```python
from build123d import *

# Parameters (mm, degrees)
SKETCH1_R           = 28
BOSS_EXTRUDE1_DEPTH = 55
CUT_EXTRUDE1_DEPTH  = 35
SKETCH3_R           = 28
SKETCH3_R_2         = 20
BOSS_EXTRUDE2_DEPTH = 35
SKETCH4_R           = 29
BOSS_EXTRUDE3_DEPTH = 87.5


with BuildPart() as part:
    # Sketch1 → Boss-Extrude1 (new, symmetric)
    with BuildSketch(Plane(origin=(0, 0, 0), x_dir=(0, 0, -1), z_dir=(1, 0, 0))):
        with BuildLine():
            ThreePointArc((1633.779443993, -91.870179926), (1388.538518192, -287.439228591), (1079.911873115, -343.474560585))
            ThreePointArc((1079.911873115, -343.474560585), (1044.034822803, -322.026545424), (1040.331298925, -280.391656157))
            ThreePointArc((1040.331298925, -280.391656157), (1037.457004109, -237.066241511), (1001.77399927, -212.326065873))
            Line((1001.77399927, -212.326065873), (-8.291026647, -52.347482052))
            ThreePointArc((-8.291026647, -52.347482052), (-52.836618688, 4.158332074), (0, 53))
            Line((0, 53), (1402, 53))
            Line((1402, 53), (1609.372117166, -14))
            ThreePointArc((1609.372117166, -14), (1641.711266017, -46.623901593), (1633.779443993, -91.870179926))
        make_face()
        with Locations((1373, 19)):
            Circle(SKETCH1_R, mode=Mode.SUBTRACT)
    extrude(amount=BOSS_EXTRUDE1_DEPTH, both=True)

    # Sketch2 → Cut-Extrude1 (cut, symmetric)
    with BuildSketch(Plane(origin=(0, 0, 0), x_dir=(0, 0, -1), z_dir=(1, 0, 0))):
        with BuildLine():
            Line((1462.900269506, 33.323690028), (1249.391694757, -251.544855987))
            Line((1249.391694757, -251.544855987), (1001.77399927, -212.326065873))
            ThreePointArc((1001.77399927, -212.326065873), (1037.457004109, -237.066241511), (1040.331298925, -280.391656157))
            ThreePointArc((1040.331298925, -280.391656157), (1044.034822803, -322.026545424), (1079.911873115, -343.474560585))
            ThreePointArc((1079.911873115, -343.474560585), (1388.538518192, -287.439228591), (1633.779443993, -91.870179926))
            ThreePointArc((1633.779443993, -91.870179926), (1641.711266017, -46.623901593), (1609.372117166, -14))
            Line((1609.372117166, -14), (1462.900269506, 33.323690028))
        make_face()
    extrude(amount=CUT_EXTRUDE1_DEPTH, both=True, mode=Mode.SUBTRACT)

    # Sketch3 → Boss-Extrude2 (add, symmetric)
    with BuildSketch(Plane(origin=(0, 0, 0), x_dir=(0, 0, -1), z_dir=(1, 0, 0))):
        with Locations((1594, -61.578335551)):
            Circle(SKETCH3_R)
        with Locations((1083, -297.578335551)):
            Circle(SKETCH3_R_2)
    extrude(amount=BOSS_EXTRUDE2_DEPTH, both=True)

    # Sketch4 → Boss-Extrude3 (add, symmetric)
    with BuildSketch(Plane(origin=(0, 0, 0), x_dir=(0, 0, -1), z_dir=(1, 0, 0))):
        Circle(SKETCH4_R)
        with Locations((157, -14)):
            Circle(SKETCH4_R)
    extrude(amount=BOSS_EXTRUDE3_DEPTH, both=True)


solid = part.part
```
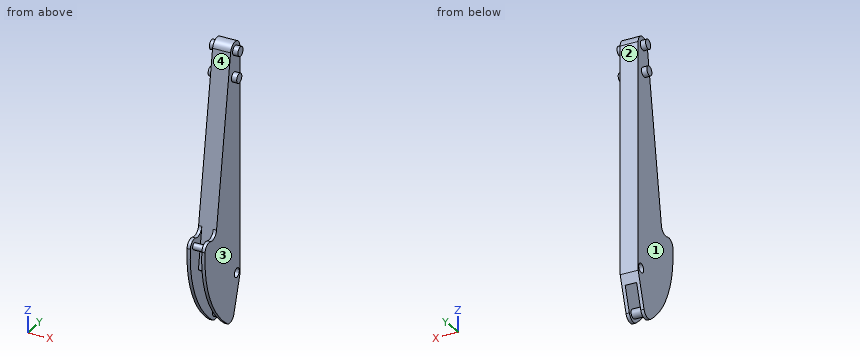
Source: CAD feature listing. Evaluate the final solid. Frame: model axes, mm. Face numbers are marked on the shaded views. Give positions to 0.01 mm unless a question says otherwise; leave off trailing zeros. Loops run counter-clockwise (first coordinate to the right, second up) from the corner with the lowest first, then second, coordinate; pieces in that order, holes last. Notation, with made-up numbers: (11.25, 51) - (55.25, 51) arc R18 ccw to (55.25, 59) - close; hole circle Ø11 at (66, 41). An arc over 180 degrees is marked (long way). Use CSV: the item, a comma, the result in double quotes.
1) Cut plane D-D (z = -157). Output: boundary loops of the cut face in (x, y).
Worked out:
outline,"(-87.5, -43) - (-55, -43) - (-55, -78.53) - (55, -78.53) - (55, -43) - (87.5, -43) - (87.5, 15) - (55, 15) - (55, 53) - (-55, 53) - (-55, 15) - (-87.5, 15) - close"
2) Cut plane B-B (x = -73). Output: boundary loops of the cut face in (y, z).
Worked out:
outline,"circle Ø58 at (-14, -157); circle Ø58 at (0, 0)"
3) Mould query, pull axis X, two halves, no side actions, for the marked faces 1, 2, 3 and 4. Classes: +X half, -X half, draft (parallel to the pull), parting line (faces both ways), or undercut.
Worked out:
face 1,"-X half"
face 2,"draft"
face 3,"+X half"
face 4,"undercut"
4) Line query: line 1 (X direction, y = -261, z = -1265); line 2 (Y direction, x = 11, z = -1373); line 3 (X direction, y = -67.5, z = -224). Output: solid intervals per line, ascending.
Worked out:
line 1,"x = -55 to -35, 35 to 55"
line 2,"y = -86.62 to -9, 47 to 53"
line 3,"x = -55 to 55"
5) Pin query (flat end, axial travel): P1, Ø5, axis at x = -42, y = -28, coming from the -Z side; P2, Ø1.5, axis at x = -12, y = -49.5, coming from the +Z side; P3, Ø3, axis at x = 35.5, y = -192, coming from the -Z side. Return the tip coordinate at first contact, or that it passes through.
Worked out:
P1,"stops at z = -1633.17"
P2,"stops at z = 20.8"
P3,"stops at z = -1540.66"
6) Cut plane A-A (x = 2). Output: boundary loops of the cut face in (y, z).
Worked out:
outline,"circle Ø40 at (-297.58, -1083); (-251.54, -1249.39) - (33.32, -1462.9) - (53, -1402) - (53, 0) arc R53 ccw to (-52.35, 8.29) - close; circle Ø56 at (-61.58, -1594); hole circle Ø56 at (19, -1373)"
7) Cut plane C-C (z = -1373). Output: boundary loops of the cut face in (x, y).
Worked out:
outline,"(-55, -294.25) - (-35, -294.25) - (-35, -86.62) - (35, -86.62) - (35, -294.25) - (55, -294.25) - (55, -9) - (-55, -9) - close; (-55, 47) - (55, 47) - (55, 53) - (-55, 53) - close"
